```python
from build123d import *

# Parameters (mm, degrees)
SKETCH_1_W      = 150
SKETCH_1_H      = 490
SKETCH_1_R      = 3.5
SKETCH_1_R_2    = 36.5
SKETCH_1_R_3    = 3.25
EXTRUDE_1_DEPTH = 20
FILLET_2_R      = 20


with BuildPart() as part:
    # Sketch 1 → Extrude 1 (new body)
    with BuildSketch(Plane.XY):
        with Locations((25, 0)):
            Rectangle(SKETCH_1_W, SKETCH_1_H)
        with Locations((-28, 215)):
            Circle(SKETCH_1_R, mode=Mode.SUBTRACT)
        with Locations((28, 215)):
            Circle(SKETCH_1_R, mode=Mode.SUBTRACT)
        with Locations((28, -215)):
            Circle(SKETCH_1_R, mode=Mode.SUBTRACT)
        with Locations((-28, -215)):
            Circle(SKETCH_1_R, mode=Mode.SUBTRACT)
        Circle(SKETCH_1_R_2, mode=Mode.SUBTRACT)
        with Locations((-34.85, 34.85)):
            Circle(SKETCH_1_R_3, mode=Mode.SUBTRACT)
        with Locations((34.85, 34.85)):
            Circle(SKETCH_1_R_3, mode=Mode.SUBTRACT)
        with Locations((34.85, -34.85)):
            Circle(SKETCH_1_R_3, mode=Mode.SUBTRACT)
        with Locations((-34.85, -34.85)):
            Circle(SKETCH_1_R_3, mode=Mode.SUBTRACT)
    extrude(amount=EXTRUDE_1_DEPTH)

    # Fillet 2
    fillet_2_edges = [part.edges().sort_by_distance(p)[0] for p in [
        (-50, -245, 10),
        (-50, 245, 10),
    ]]
    fillet(fillet_2_edges, radius=FILLET_2_R)


solid = part.part
```
Part model, mm, in its own coordinate system. Round coordinates to 2 decimals unless told otherwise and drop trailing zeros. Loops run counter-clockwise (first coordinate to the right, second up) from the corner with the lowest first, then second, coordinate; pieces in that order, holes last. Notation, with made-up numbers: (75, 82.5) -> (81, 82.5) arc R9 cw to (81, 91.5) -> close; hole circle Ø3 at (37, 59.5). An arc over 180 degrees is marked (long way). Use a Markdown table: item, result.
1) Pull direction Y, two halves, no side cores. Call faces 1 (the cylindrical face through (-7.912, -35.632, 9.86)), 2 (the cylindrical face through (-44.297, -238.986, 10.14)), 3 (the flat face through (34, 245, 10)), 4 (the flat face through (41, 3, 0)): pulls with the +Y half, pulls with the -Y half, needs draft (parallel to the pull), parting line crosses it, or undercut.
The answers:
| item | result |
|---|---|
| face 1 | undercut |
| face 2 | pulls with the -Y half |
| face 3 | pulls with the +Y half |
| face 4 | needs draft |
2) Cut at B-B, the plane x = 0. List the corners of the cut face in (y, z), and give its area (3 significant figures).
The answers:
| item | result |
|---|---|
| outline | (-245, 0) -> (-36.5, 0) -> (-36.5, 20) -> (-245, 20) -> close; (36.5, 0) -> (245, 0) -> (245, 20) -> (36.5, 20) -> close |
| area | 8,340 mm2 |
3) Cut at A-A, the plane z = 11.25. State how many separate pieces and enclosed holes the cut face has, and give its area (3 significant figures).
The answers:
| item | result |
|---|---|
| separate pieces | 1 |
| enclosed holes | 9 |
| area | 68,900 mm2 |
4) Probe line 1 (X direction, y = -215, z = 4.5); line 2 (X direction, y = -213, z = 4); line 3 (Y direction, x = -28, z = 4.5). List the from-to ranges inside material, lowest first. Write a range as [from, to].
The answers:
| item | result |
|---|---|
| line 1 | x = [-50, -31.5], [-24.5, 24.5], [31.5, 100] |
| line 2 | x = [-50, -30.87], [-25.13, 25.13], [30.87, 100] |
| line 3 | y = [-245, -218.5], [-211.5, -23.41], [23.41, 211.5], [218.5, 245] |
5) Drop flat-ended pins along their axis: pin 1 Ø6.5 at (x, y) = (-28, 215) entering from +Z; pin 2 Ø8 at (x, y) = (-28, -215) entering from +Z. Give the stop position or say it passes through.
The answers:
| item | result |
|---|---|
| pin 1 | passes through |
| pin 2 | stops at z = 20 |
